Source: CAD feature listing. Evaluate the final solid. Frame: model axes, mm. Round coordinates to 2 decimals unless told otherwise and drop trailing zeros. Loops run counter-clockwise (first coordinate to the right, second up) from the corner with the lowest first, then second, coordinate; pieces in that order, holes last. Notation, with made-up numbers: M -5,39 L 45,39 A21 ccw 45,67 Z; hole C 69,79 d9. An arc over 180 degrees is marked long. Write each question's results on one line, items separated by ' | '. Start each with the question number.
1. Section C-C on y = 72.5. Output: boundary loops of the cut face in (x, z).
2. Ray query, line 1 (Y direction, x = 0, z = 0.8); line 2 (Y direction, x = -175, z = 1.5); line 3 (Y direction, x = -168, z = 1). Return the intervals inside material, ascending.
3. Draft query along X for faces 1 (the flat face through (-5, 132, 0)), 2 (the cylindrical face through (-0.867, -3.905, 0.986)), 3 (the cylindrical face through (8.805, 184.062, 0.986)), 4 (the cylindrical face through (-172.85, 178.447, 0.986)). Return one class per face: released by +X, released by -X, zero draft, split by the parting line, or undercut.
4. Contact query for a flat-ended pin moving along its axis: pin 1 Ø0.6 at (y, z) = (110, 1) entering from -X. Output: stop coordinate, or through.
5. Section B-B on x = -99.5. Output: boundary loops of the cut face in (y, z).
6. Section A-A on z = 1.25. Give the number of separate pieces and of enclosed holes in the cut face, and give its area (3 significant figures).
from build123d import *

# Parameters (mm, degrees)
SKETCH_1_R      = 4
SKETCH_1_R_2    = 1.5
EXTRUDE_2_DEPTH = 2


with BuildPart() as part:
    # 草图1 → 凸台-拉伸2 (new body)
    with BuildSketch(Plane.XY):
        with BuildLine():
            Line((-12.585683816, 0), (-12.585683816, 162.5))
            Line((-12.585683816, 162.5), (-175, 162.5))
            ThreePointArc((-175, 162.5), (-187.573970324, 175.073970324), (-175, 187.647940648))
            Line((-175, 187.647940648), (0.011713493, 187.647940648))
            ThreePointArc((0.011713493, 187.647940648), (8.902853175, 183.965110006), (12.585683816, 175.073970324))
            Line((12.585683816, 175.073970324), (12.585683816, 0))
            ThreePointArc((12.585683816, 0), (0, -12.585683816), (-12.585683816, 0))
        make_face()
        Circle(SKETCH_1_R, mode=Mode.SUBTRACT)
        with Locations((-175, 175.073970324)):
            Circle(SKETCH_1_R, mode=Mode.SUBTRACT)
        with Locations((-175, 182.073970324)):
            Circle(SKETCH_1_R_2, mode=Mode.SUBTRACT)
        with Locations((-168, 175.073970324)):
            Circle(SKETCH_1_R_2, mode=Mode.SUBTRACT)
        with Locations((-175, 168.073970324)):
            Circle(SKETCH_1_R_2, mode=Mode.SUBTRACT)
        with Locations((-182, 175.073970324)):
            Circle(SKETCH_1_R_2, mode=Mode.SUBTRACT)
        with Locations((0, 130)):
            Circle(SKETCH_1_R_2, mode=Mode.SUBTRACT)
        with Locations((-45, 175.073970324)):
            Circle(SKETCH_1_R_2, mode=Mode.SUBTRACT)
        with Locations((4.949747468, 4.949747468)):
            Circle(SKETCH_1_R_2, mode=Mode.SUBTRACT)
        with Locations((4.949747468, -4.949747468)):
            Circle(SKETCH_1_R_2, mode=Mode.SUBTRACT)
        with Locations((-4.949747468, -4.949747468)):
            Circle(SKETCH_1_R_2, mode=Mode.SUBTRACT)
        with Locations((-4.949747468, 4.949747468)):
            Circle(SKETCH_1_R_2, mode=Mode.SUBTRACT)
    extrude(amount=EXTRUDE_2_DEPTH)


solid = part.part
Taken from the geometry:
1) outline: M -12.59,0 L 12.59,0 L 12.59,2 L -12.59,2 Z
2) line 1: -12.59 to -4, 4 to 128.5, 131.5 to 187.65 | line 2: 162.5 to 166.57, 169.57 to 171.07, 179.07 to 180.57, 183.57 to 187.65 | line 3: 162.5 to 173.57, 176.57 to 187.65
3) face 1: zero draft | face 2: undercut | face 3: released by +X | face 4: undercut
4) pin 1: x = -12.59
5) outline: M 162.5,0 L 187.65,0 L 187.65,2 L 162.5,2 Z
6) separate pieces: 1 | enclosed holes: 12 | area: 9,100 mm^2
